Build history of the part. All positions in model axes, mm. Give positions to 0.01 mm unless a question says otherwise; leave off trailing zeros. Order: outer loops, then holes, each group sorted by start corner. A loop starts at its lowest first (then second) coordinate and runs counter-clockwise, first axis right, second up. Notation, with made-up numbers: (28.25, -24.75) -> (76.25, -24.75) arc R31 ccw to (76.25, 6.25) -> close; hole circle Ø11 at (30, -10). An arc over 180 degrees is marked (long way). Use a Markdown table: item, result. Add a question column.
```python
from build123d import *

# Parameters (mm, degrees)
F0_R     = 7.5
F1_DEPTH = 500
F2_SIZE  = 2
F3_R     = 4
F4_DEPTH = 10


with BuildPart() as f1:
    # F0 (on Top) → F1 (new body)
    with BuildSketch(Plane.XY):
        Circle(F0_R)
    extrude(amount=F1_DEPTH)

    # F2
    f2_edges = [f1.edges().sort_by_distance(p)[0] for p in [
        (-7.5, 0, 0),
        (-7.5, 0, 500),
    ]]
    chamfer(f2_edges, length=F2_SIZE)

    # F3 (on Front) → F4 (cut, symmetric)
    with BuildSketch(Plane.XZ):
        with Locations((0, 10)):
            Circle(F3_R)
        with Locations((0, 120)):
            Circle(F3_R)
    extrude(amount=F4_DEPTH, both=True, mode=Mode.SUBTRACT)


solid = f1.part
```
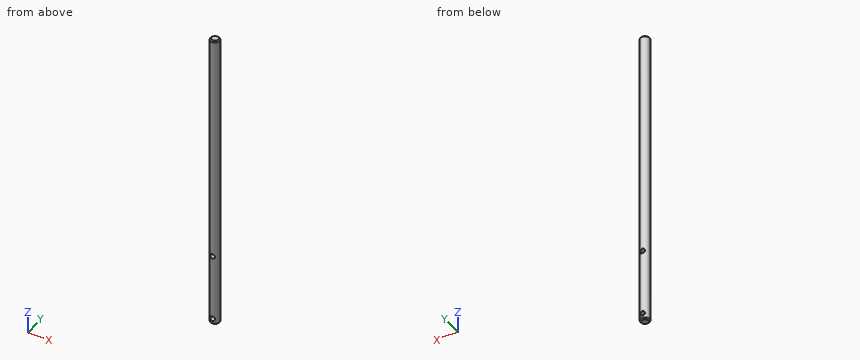
(1) Wall check: probe 1 along Z at (x, y) = (0, -3.25); probe 2 along X at (y, z) = (-0.75, 120); probe 3 along Y at (x, z) = (5, 397.5). Give the ranges that are in metal, low to high.
(2) Band-saw the part on A-A on x = 0. Give the cut face in (y, z).
(3) Band-saw the part on B-B on z = 202. Give the cut face in (x, y).
(4) Pin check, flat tips, straight feed: pin 1 Ø6.5 at (x, z) = (0, 10) entering from -Y; pin 2 Ø5 at (x, z) = (-6, 248.5) entering from -Y. Stop position of each tip, or through.
Response:
| question | item | result |
|---|---|---|
| 1 | probe 1 | z = 0 to 6, 14 to 116, 124 to 500 |
| 1 | probe 2 | x = -7.46 to -4, 4 to 7.46 |
| 1 | probe 3 | y = -5.59 to 5.59 |
| 2 | outline | (-7.5, 2) -> (-5.5, 0) -> (5.5, 0) -> (7.5, 2) -> (7.5, 6) -> (-7.5, 6) -> close; (-7.5, 14) -> (7.5, 14) -> (7.5, 116) -> (-7.5, 116) -> close; (-7.5, 124) -> (7.5, 124) -> (7.5, 498) -> (5.5, 500) -> (-5.5, 500) -> (-7.5, 498) -> close |
| 3 | outline | circle Ø15 at (0, 0) |
| 4 | pin 1 | passes through |
| 4 | pin 2 | stops at y = -6.63 |
